The model under review builds one solid part; all positions refer to its coordinate system, in mm. A direction names the side the tool comes from. Give positions to 0.01 mm unless a question says otherwise; leave off trailing zeros. Order: outer loops, then holes, each group sorted by start corner. A loop starts at its lowest first (then second) coordinate and runs counter-clockwise, first axis right, second up. Notation, with made-up numbers: (38.5, -8.5) -> (70.5, -8.5) arc R6 cw to (70.5, 1.5) -> close; hole circle Ø7 at (64, -39.75). An arc over 180 degrees is marked (long way). Use one line per item in the form item = value.
```python
from build123d import *

# Parameters (mm, degrees)
SKETCH3_R          = 2
CUT_EXTRUDE1_DEPTH = 93.838569571
SKETCH5_R          = 1.5
CUT_EXTRUDE2_DEPTH = 94.305948363
CIRPATTERN1_COUNT  = 4


with BuildPart() as part:
    # Sketch2 → Revolve1 (revolve)
    with BuildSketch(Plane.XY, mode=Mode.PRIVATE) as revolve1_sk:
        Polygon((30.6, 16), (30.6, 0), (65, 0), (65, 3), (33.6, 3), (33.6, 16), align=None)
    revolve(revolve1_sk.sketch.rotate(Axis((0, 31.868523677, 0), (0, -1, 0)), 90), axis=Axis((0, 31.868523677, 0), (0, -1, 0)))

    # Sketch3 → Cut-Extrude1 (cut, through all)
    with BuildSketch(Plane(origin=(0, 3, 0), x_dir=(1, 0, 0), z_dir=(0, 1, 0))):
        with Locations(Location((0, 50, 0), (0, 0, 270))):
            Circle(SKETCH3_R)
        with Locations(Location((50, 0, 0), (0, 0, 270))):
            Circle(SKETCH3_R)
        with Locations(Location((0, -50, 0), (0, 0, 270))):
            Circle(SKETCH3_R)
        with Locations(Location((-50, 0, 0), (0, 0, 270))):
            Circle(SKETCH3_R)
    extrude(amount=-CUT_EXTRUDE1_DEPTH, mode=Mode.SUBTRACT)

    # Sketch5 → Cut-Extrude2 (cut, through all)
    with BuildSketch(Plane(origin=(0, 0, 0), x_dir=(0, 1, 0), z_dir=(0.7071067811865488, 0, 0.7071067811865464))):
        with Locations(Location((8, 0, 0), (0, 0, 270))):
            Circle(SKETCH5_R)
    cut_extrude2 = extrude(amount=-CUT_EXTRUDE2_DEPTH, mode=Mode.SUBTRACT)

    # CirPattern1: Cut-Extrude2 ×4 about axis
    cirpattern1_axis = Axis((0, 31.868523677, 0), (0, 1, 0))
    for i in range(1, CIRPATTERN1_COUNT):
        add(cut_extrude2.rotate(cirpattern1_axis, i * 360 / CIRPATTERN1_COUNT), mode=Mode.SUBTRACT)


solid = part.part
```
1. Add section B-B on x = 0. Give the boundary of the cut face in (y, z), then the cut area to 3 significant figures.
Values:
outline = (0, -65) -> (3, -65) -> (3, -52) -> (0, -52) -> close; (0, -48) -> (3, -48) -> (3, -33.6) -> (16, -33.6) -> (16, -30.6) -> (0, -30.6) -> close; (0, 30.6) -> (16, 30.6) -> (16, 33.6) -> (3, 33.6) -> (3, 48) -> (0, 48) -> close; (0, 52) -> (3, 52) -> (3, 65) -> (0, 65) -> close
area = 260 mm^2
2. Add section C-C on x = 15. Give the boundary of the cut face in (y, z).
Values:
outline = (0, -63.25) -> (3, -63.25) -> (3, -30.07) -> (16, -30.07) -> (16, -26.67) -> (0, -26.67) -> close; (0, 26.67) -> (16, 26.67) -> (16, 30.07) -> (3, 30.07) -> (3, 63.25) -> (0, 63.25) -> close
3. Add section D-D on z = 16. Give the boundary of the cut face in (x, y).
Values:
outline = (-63, 0) -> (-26.08, 0) -> (-26.08, 16) -> (-29.55, 16) -> (-29.55, 3) -> (-63, 3) -> close; (26.08, 0) -> (63, 0) -> (63, 3) -> (29.55, 3) -> (29.55, 16) -> (26.08, 16) -> close
4. For L1, parallel to X at y = 2.3, z = 0; L2, parallel to X at y = 12.5, z = 0; L3, parallel to Y at x = 57, z = -6.5, list the stretches that pass through material, from the lowest coordinate up.
Values:
L1 = -65 to -52, -48 to -30.6, 30.6 to 48, 52 to 65
L2 = -33.6 to -30.6, 30.6 to 33.6
L3 = 0 to 3
5. Tool access review of faces 4 (the face through (28, 3, 28)), 5 (the face through (-0.766, 1.521, 51.847)): name each direction out of +Z, -Z, +X, -X, +Y, -Y from which nothing blocks a thin tool from reaching the whole face with its end or side.
Values:
face_4 = +Y
face_5 = +Y, -Y
6. Add section A-A on z = 0. Give the boundary of the cut face in (x, y).
Values:
outline = (-65, 0) -> (-52, 0) -> (-52, 3) -> (-65, 3) -> close; (-48, 0) -> (-30.6, 0) -> (-30.6, 16) -> (-33.6, 16) -> (-33.6, 3) -> (-48, 3) -> close; (30.6, 0) -> (48, 0) -> (48, 3) -> (33.6, 3) -> (33.6, 16) -> (30.6, 16) -> close; (52, 0) -> (65, 0) -> (65, 3) -> (52, 3) -> close
7. For pin 1 Ø4.5 at (x, z) = (-50, 0) entering from +Y; pin 2 Ø2 at (x, y) = (19, 4.5) entering from -Z; pin 3 Ø8 at (x, y) = (26, 11.5) entering from -Z; pin 4 Ø2 at (x, z) = (-37, -7.5) entering from -Y, all flat-tipped, find the tip position at first contact; note any pin that passes through.
Values:
pin_1 = 3
pin_2 = -28.37
pin_3 = -25.4
pin_4 = 0
8. The part is to be moulded in two halves that separate along Z. For faces 1 (the face through (-8, 16, 30)), 2 (the face through (-19.52, 1.52, 62)), 3 (the face through (27.147, 7.888, 14.12)), say which applies: +Z half, -Z half, draft (parallel to the pull), parting line (faces both ways), or undercut.
Values:
face_1 = draft
face_2 = parting line
face_3 = undercut
